from build123d import *

# Parameters (mm, degrees)
SKETCH_1_W          = 50
SKETCH_1_H          = 30
EXTRUDE_1_DEPTH     = 7
SKETCH_2_W          = 10
SKETCH_2_H          = 25
CUT_EXTRUDE_1_DEPTH = 4
SKETCH_4_R          = 1.6
CUT_EXTRUDE_3_DEPTH = 30.983328701
SKETCH_5_R          = 3
CUT_EXTRUDE_4_DEPTH = 3
SKETCH_6_R          = 1.5
CUT_EXTRUDE_5_DEPTH = 30.983328701
SKETCH_7_W          = 13
SKETCH_7_H          = 14
EXTRUDE_6_DEPTH     = 11
SKETCH_8_R          = 1.5
CUT_EXTRUDE_6_DEPTH = 32.160872902
SKETCH_9_R          = 1.5
CUT_EXTRUDE_7_DEPTH = 35.263683398
FILLET_1_R          = 2
SKETCH_10_W         = 4
SKETCH_10_H         = 10
CUT_EXTRUDE_8_DEPTH = 4
FILLET_2_R          = 1
FILLET_3_R          = 1


with BuildPart() as part:
    # Эскиз1 → Бобышка-Вытянуть1 (new body)
    with BuildSketch(Plane(origin=(0, 0, 0), x_dir=(1, 0, 0), z_dir=(0, 1, 0))):
        Rectangle(SKETCH_1_W, SKETCH_1_H)
    extrude(amount=EXTRUDE_1_DEPTH)

    # Эскиз2 → Вырез-Вытянуть1 (cut)
    with BuildSketch(Plane(origin=(0, 7, 0), x_dir=(1, 0, 0), z_dir=(0, 1, 0))):
        with Locations((-12.5, -2.5)):
            Rectangle(SKETCH_2_W, SKETCH_2_H)
        with Locations((12.5, -2.5)):
            Rectangle(SKETCH_2_W, SKETCH_2_H)
    extrude(amount=-CUT_EXTRUDE_1_DEPTH, mode=Mode.SUBTRACT)

    # Эскиз4 → Вырез-Вытянуть3 (cut, through all)
    with BuildSketch(Plane(origin=(0, 7, 0), x_dir=(1, 0, 0), z_dir=(0, 1, 0))):
        with Locations(Location((0, 5, 0), (0, 0, 270))):
            Circle(SKETCH_4_R)
    extrude(amount=-CUT_EXTRUDE_3_DEPTH, mode=Mode.SUBTRACT)

    # Эскиз5 → Вырез-Вытянуть4 (cut)
    with BuildSketch(Plane.XZ):
        with Locations(Location((0, -5, 0), (0, 0, 270))):
            Circle(SKETCH_5_R)
    extrude(amount=-CUT_EXTRUDE_4_DEPTH, mode=Mode.SUBTRACT)

    # Эскиз6 → Вырез-Вытянуть5 (cut, through all)
    with BuildSketch(Plane(origin=(0, 7, 0), x_dir=(1, 0, 0), z_dir=(0, 1, 0))):
        with Locations(Location((-21.25, 0, 0), (0, 0, 270))):
            Circle(SKETCH_6_R)
        with Locations(Location((0, 12.5, 0), (0, 0, 270))):
            Circle(SKETCH_6_R)
        with Locations(Location((21.25, 0, 0), (0, 0, 270))):
            Circle(SKETCH_6_R)
        with Locations(Location((0, -7.5, 0), (0, 0, 270))):
            Circle(SKETCH_6_R)
    extrude(amount=-CUT_EXTRUDE_5_DEPTH, mode=Mode.SUBTRACT)

    # Эскиз7 → Бобышка-Вытянуть6 (add)
    with BuildSketch(Plane(origin=(0, 7, 0), x_dir=(1, 0, 0), z_dir=(0, 1, 0))):
        Polygon((-25, 15), (25, 15), (25, -15), (18.5, -15), (18.5, 10.5), (-18.5, 10.5), (-18.5, -15), (-25, -15), align=None)
        with Locations((0, -8)):
            Rectangle(SKETCH_7_W, SKETCH_7_H)
    extrude(amount=EXTRUDE_6_DEPTH)

    # Эскиз8 → Вырез-Вытянуть6 (cut, through all)
    with BuildSketch(Plane.XZ.offset(-7)):
        with Locations(Location((21.25, 0, 0), (0, 0, 90))):
            Circle(SKETCH_8_R)
        with Locations(Location((0, 7.5, 0), (0, 0, 90))):
            Circle(SKETCH_8_R)
        with Locations(Location((-21.25, 0, 0), (0, 0, 90))):
            Circle(SKETCH_8_R)
        with Locations(Location((0, -12.5, 0), (0, 0, 90))):
            Circle(SKETCH_8_R)
    extrude(amount=-CUT_EXTRUDE_6_DEPTH, mode=Mode.SUBTRACT)

    # Эскиз9 → Вырез-Вытянуть7 (cut, through all)
    with BuildSketch(Plane(origin=(0, 18, 0), x_dir=(1, 0, 0), z_dir=(0, 1, 0))):
        with Locations(Location((-21.25, 10, 0), (0, 0, 270))):
            Circle(SKETCH_9_R)
        with Locations(Location((21.25, 10, 0), (0, 0, 270))):
            Circle(SKETCH_9_R)
        with Locations(Location((21.25, -10, 0), (0, 0, 270))):
            Circle(SKETCH_9_R)
        with Locations(Location((-21.25, -10, 0), (0, 0, 270))):
            Circle(SKETCH_9_R)
    extrude(amount=-CUT_EXTRUDE_7_DEPTH, mode=Mode.SUBTRACT)

    # Скругление1
    # the kernel refuses this fillet: 2 mm, written as the material it takes off along each edge
    with BuildSketch(Plane(origin=(-23, 2, -13), x_dir=(0, -1, 0), z_dir=(-1, 0, 0))) as fillet_1_piece_1_section:
        Polygon((0, 0), (FILLET_1_R, 0), (FILLET_1_R, -FILLET_1_R), (0, -FILLET_1_R), align=None)
    fillet_1_piece_1 = extrude(amount=FILLET_1_R, mode=Mode.PRIVATE)
    fillet_1_piece_1 = fillet_1_piece_1 - Plane(origin=(-23, 2, -13), x_dir=(0, 0.7071067811865475, 0.7071067811865475), z_dir=(-1, 0, 0)) * Sphere(FILLET_1_R, mode=Mode.PRIVATE)
    add(fillet_1_piece_1, mode=Mode.SUBTRACT)
    with BuildSketch(Plane(origin=(23, 2, -13), x_dir=(1, 0, 0), z_dir=(0, -1, 0))) as fillet_1_piece_2_section:
        Polygon((0, 0), (FILLET_1_R, 0), (FILLET_1_R, -FILLET_1_R), (0, -FILLET_1_R), align=None)
    fillet_1_piece_2 = extrude(amount=FILLET_1_R, mode=Mode.PRIVATE)
    fillet_1_piece_2 = fillet_1_piece_2 - Plane(origin=(23, 2, -13), x_dir=(-0.7071067811865474, 0, 0.7071067811865477), z_dir=(0, -1, 0)) * Sphere(FILLET_1_R, mode=Mode.PRIVATE)
    add(fillet_1_piece_2, mode=Mode.SUBTRACT)
    with BuildSketch(Plane(origin=(23, 2, 13), x_dir=(0, -1, 0), z_dir=(0, 0, 1))) as fillet_1_piece_3_section:
        Polygon((0, 0), (FILLET_1_R, 0), (FILLET_1_R, FILLET_1_R), (0, FILLET_1_R), align=None)
    fillet_1_piece_3 = extrude(amount=FILLET_1_R, mode=Mode.PRIVATE)
    fillet_1_piece_3 = fillet_1_piece_3 - Plane(origin=(23, 2, 13), x_dir=(-0.7071067811865475, 0.7071067811865475, 0), z_dir=(0, 0, 1)) * Sphere(FILLET_1_R, mode=Mode.PRIVATE)
    add(fillet_1_piece_3, mode=Mode.SUBTRACT)
    with BuildSketch(Plane(origin=(-23, 2, 13), x_dir=(0, -1, 0), z_dir=(0, 0, 1))) as fillet_1_piece_4_section:
        Polygon((0, 0), (FILLET_1_R, 0), (FILLET_1_R, -FILLET_1_R), (0, -FILLET_1_R), align=None)
    fillet_1_piece_4 = extrude(amount=FILLET_1_R, mode=Mode.PRIVATE)
    fillet_1_piece_4 = fillet_1_piece_4 - Plane(origin=(-23, 2, 13), x_dir=(0.7071067811865475, 0.7071067811865475, 0), z_dir=(0, 0, 1)) * Sphere(FILLET_1_R, mode=Mode.PRIVATE)
    add(fillet_1_piece_4, mode=Mode.SUBTRACT)
    with BuildSketch(Plane(origin=(-23, 0, -15), x_dir=(0, 0, 1), z_dir=(1, 0, 0))) as fillet_1_piece_5:
        with BuildLine():
            CenterArc((FILLET_1_R, -FILLET_1_R), FILLET_1_R, 90, 90)
            Line((0, -FILLET_1_R), (0, 0))
            Line((0, 0), (FILLET_1_R, 0))
        make_face()
    extrude(amount=46, mode=Mode.SUBTRACT)
    with BuildSketch(Plane(origin=(25, 0, -13), x_dir=(-1, 0, 0), z_dir=(0, 0, 1)), Plane(origin=(-25, 0, 13), x_dir=(1, 0, 0), z_dir=(0, 0, -1))) as fillet_1_piece_6:
        with BuildLine():
            CenterArc((FILLET_1_R, -FILLET_1_R), FILLET_1_R, 90, 90)
            Line((0, -FILLET_1_R), (0, 0))
            Line((0, 0), (FILLET_1_R, 0))
        make_face()
    extrude(amount=26, mode=Mode.SUBTRACT)
    with BuildSketch(Plane(origin=(23, 0, 15), x_dir=(0, 1, 0), z_dir=(-1, 0, 0))) as fillet_1_piece_7:
        with BuildLine():
            CenterArc((FILLET_1_R, FILLET_1_R), FILLET_1_R, 180, 90)
            Line((0, FILLET_1_R), (0, 0))
            Line((0, 0), (FILLET_1_R, 0))
        make_face()
    extrude(amount=46, mode=Mode.SUBTRACT)
    with BuildSketch(Plane(origin=(-25, 23, -15), x_dir=(0, 0, 1), z_dir=(0, -1, 0)), Plane(origin=(25, 2, -15), x_dir=(0, 0, 1), z_dir=(0, 1, 0)), Plane(origin=(25, 2, 15), x_dir=(-1, 0, 0), z_dir=(0, 1, 0)), Plane(origin=(-25, 23, 15), x_dir=(1, 0, 0), z_dir=(0, -1, 0))) as fillet_1_piece_8:
        with BuildLine():
            CenterArc((FILLET_1_R, -FILLET_1_R), FILLET_1_R, 90, 90)
            Line((0, -FILLET_1_R), (0, 0))
            Line((0, 0), (FILLET_1_R, 0))
        make_face()
    extrude(amount=21, mode=Mode.SUBTRACT)

    # Эскиз10 → Вырез-Вытянуть8 (cut)
    with BuildSketch(Plane(origin=(0, 7, 0), x_dir=(1, 0, 0), z_dir=(0, 1, 0))):
        with Locations((-5.5, 5)):
            Rectangle(SKETCH_10_W, SKETCH_10_H)
        with Locations((5.5, 5)):
            Rectangle(SKETCH_10_W, SKETCH_10_H)
    extrude(amount=-CUT_EXTRUDE_8_DEPTH, mode=Mode.SUBTRACT)

    # Скругление2
    fillet_2_edges = [part.edges().sort_by_distance(p)[0] for p in [
        (-7.5, 5, 0),
        (-3.5, 5, -10),
        (-3.5, 5, 0),
        (7.5, 5, 0),
        (3.5, 5, 0),
        (3.5, 5, -10),
    ]]
    fillet(fillet_2_edges, radius=FILLET_2_R)

    # Скругление3
    fillet_3_edges = [part.edges().sort_by_distance(p)[0] for p in [
        (17.5, 5, -10),
        (17.5, 5, 15),
        (7.5, 5, 15),
        (-7.5, 5, 15),
        (-17.5, 5, 15),
        (-17.5, 5, -10),
    ]]
    fillet(fillet_3_edges, radius=FILLET_3_R)


solid = part.part
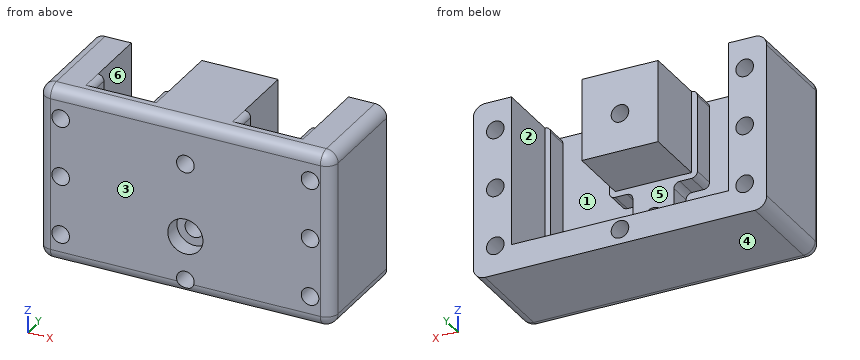
Here's how the part is built. I have some questions about the finished solid (model axes, mm). Face numbers are marked on the shaded views. A direction names the side the tool comes from. Round coordinates to 2 decimals unless told otherwise and drop trailing zeros. Order: outer loops, then holes, each group sorted by start corner. A loop starts at its lowest first (then second) coordinate and runs counter-clockwise, first axis right, second up. Notation, with made-up numbers: M 19.25,-10.75 L 62.25,-10.75 A20 ccw 62.25,2.25 Z; hole C 56.5,65 d3. An arc over 180 degrees is marked long. Return JSON: item names as keys, results as strings. Group by question number.
1. If we mould it in two halves opening along Z, with no side actions, what happens to the marked faces 4, 5 and 6? For each: pulls with the +Z half, pulls with the -Z half, needs draft (parallel to the pull), parting line crosses it, or undercut.
2. If we section it at D-D on z = -5: List the corners of the cut face in (x, y) for me, then the cut area to 3 significant figures.
3. On a 3-axis mill with a long thin cutter (end or side, diameter ignored), from which of +Z, -Z, +X, -X, +Y, -Y can I reach the whole of each face in a straight line? I mean the marked faces 1, 2 and 3. Say none if no direction works.
4. If we section it at B-B on x = -21.25: List the corners of the cut face in (y, z) for me, then the cut area to 3 significant figures.
5. I'm going to push flat-ended pins straight in: pin 1 Ø4 at (x, y) = (-9, 15.5) entering from +Z; pin 2 Ø1.5 at (x, z) = (15, 9.5) entering from +Y; pin 3 Ø5.5 at (x, z) = (0, -5) entering from +Y. Where does each tip first touch, or does it pass through?
6. Please list where these lines run through material, in increasing order: probe 1 along X at (y, z) = (8.25, 0); probe 2 along X at (y, z) = (4.5, 10); probe 3 along X at (y, z) = (13.75, -12.5).
7. If we section it at A-A on y = 11: State how many separate pieces and enclosed holes the cut face has, then the cut area to 3 significant figures.
Reply:
{
 "1": {"face 4": "pulls with the -Z half", "face 5": "undercut", "face 6": "needs draft"},
 "2": {"outline": "M -25,2 A2 ccw -23,0 L -3,0 L -3,3 L -1.6,3 L -1.6,7 L -3.5,7 L -3.5,3 L -17.5,3 L -17.5,7 L -18.5,7 L -18.5,18 L -25,18 Z; M 1.6,3 L 3,3 L 3,0 L 23,0 A2 ccw 25,2 L 25,18 L 18.5,18 L 18.5,7 L 17.5,7 L 17.5,3 L 3.5,3 L 3.5,7 L 1.6,7 Z", "area": "348 mm^2"},
 "3": {"face 1": "+Y", "face 2": "+Z, +Y", "face 3": "+Z, -Z, +X, -X, -Y"},
 "4": {"outline": "M 0,-13 A2 ccw 2,-15 L 18,-15 L 18,-11.5 L 0,-11.5 Z; M 0,-8.5 L 18,-8.5 L 18,-1.5 L 0,-1.5 Z; M 0,1.5 L 18,1.5 L 18,8.5 L 0,8.5 Z; M 0,11.5 L 18,11.5 L 18,15 L 2,15 A2 ccw 0,13 Z", "area": "376 mm^2"},
 "5": {"pin 1": "z = -10.5", "pin 2": "y = 3", "pin 3": "y = 7"},
 "6": {"probe 1": "-25 to -22.75, -19.75 to -18.5, 18.5 to 19.75, 22.75 to 25", "probe 2": "-25 to -22.75, -19.75 to -17.5, -7.5 to 7.5, 17.5 to 19.75, 22.75 to 25", "probe 3": "-25 to -1.5, 1.5 to 25"},
 "7": {"separate pieces": "2", "enclosed holes": "8", "area": "679 mm^2"}
}
